```python
from build123d import *

# Parameters (mm, degrees)
SKETCH_1_R          = 9
EXTRUDE_1_DEPTH     = 2
SKETCH_2_R          = 6.78
EXTRUDE_2_DEPTH     = 11
SKETCH_3_R          = 9
EXTRUDE_3_DEPTH     = 2
SKETCH_4_R          = 2.5
CUT_EXTRUDE_1_DEPTH = 26


with BuildPart() as part:
    # 草图1 → 凸台-拉伸1 (new body)
    with BuildSketch(Plane(origin=(0, 0, 0), x_dir=(1, 0, 0), z_dir=(0, 1, 0))):
        with Locations(Location((0, 0, 0), (0, 0, 270))):
            Circle(SKETCH_1_R)
    extrude(amount=EXTRUDE_1_DEPTH)

    # 草图2 → 凸台-拉伸2 (add)
    with BuildSketch(Plane(origin=(0, 2, 0), x_dir=(1, 0, 0), z_dir=(0, 1, 0))):
        with Locations(Location((0, 0, 0), (0, 0, 270))):
            Circle(SKETCH_2_R)
    extrude(amount=EXTRUDE_2_DEPTH)

    # 草图3 → 凸台-拉伸3 (add)
    with BuildSketch(Plane(origin=(0, 13, 0), x_dir=(1, 0, 0), z_dir=(0, 1, 0))):
        with Locations(Location((0, 0, 0), (0, 0, 270))):
            Circle(SKETCH_3_R)
    extrude(amount=EXTRUDE_3_DEPTH)

    # 草图4 → 切除-拉伸1 (cut)
    with BuildSketch(Plane(origin=(0, 15, 0), x_dir=(1, 0, 0), z_dir=(0, 1, 0))):
        with Locations(Location((0, 0, 0), (0, 0, 270))):
            Circle(SKETCH_4_R)
    extrude(amount=-CUT_EXTRUDE_1_DEPTH, mode=Mode.SUBTRACT)


solid = part.part
```
Geometry check sheet. Reference: the model listing, model coordinates, mm. A direction names the side the tool comes from. Coordinates: 2 decimals unless noted, no trailing zeros. Order: outer loops, then holes, each group sorted by start corner. A loop starts at its lowest first (then second) coordinate and runs counter-clockwise, first axis right, second up. Notation, with made-up numbers: M 6,68 L 46,68 A9 cw 46,82 Z; hole C -26,64 d3. An arc over 180 degrees is marked long. Answer as a JSON object with one key per item and string values.
Q1. Scan lines: line 1 (Y direction, x = -3.5, z = 8.25); line 2 (X direction, y = 10, z = 0); line 3 (X direction, y = 10.5, z = -1.5). Record each from-to range of solid material in increasing order.
Results are:
{"line 1": "y = 0 to 2, 13 to 15", "line 2": "x = -6.78 to -2.5, 2.5 to 6.78", "line 3": "x = -6.61 to -2, 2 to 6.61"}
Q2. Tool access check on faces 1 (the flat face through (-2, 15, 2)), 2 (the flat face through (7, 2, 1)). Record the directions out of +Z, -Z, +X, -X, +Y, -Y that give a thin tool (end or side, any length) a straight path to the whole face; none if there is none.
Results are:
{"face 1": "+Z, -Z, +X, -X, +Y", "face 2": "none"}
Q3. Cross-section at A-A on x = 0. Record the cut outline in (y, z), and give its area (3 significant figures).
Results are:
{"outline": "M 0,-9 L 2,-9 L 2,-6.78 L 13,-6.78 L 13,-9 L 15,-9 L 15,-2.5 L 0,-2.5 Z; M 0,2.5 L 15,2.5 L 15,9 L 13,9 L 13,6.78 L 2,6.78 L 2,9 L 0,9 Z", "area": "146 mm²"}
Q4. Depth check by flat-ended pin: pin 1 Ø5 at (y, z) = (4, -5) entering from +X; pin 2 Ø2 at (x, y) = (2.5, 4) entering from -Z; pin 3 Ø5 at (y, z) = (5.5, 1) entering from +X. Enter the tip coordinate at first touch or a pass-through.
Results are:
{"pin 1": "stops at x = 8.29", "pin 2": "stops at z = -6.61", "pin 3": "stops at x = 6.78"}
Q5. Cross-section at B-B on z = 0. Record the cut outline in (x, y), and give its area (3 significant figures).
Results are:
{"outline": "M -9,0 L -2.5,0 L -2.5,15 L -9,15 L -9,13 L -6.78,13 L -6.78,2 L -9,2 Z; M 2.5,0 L 9,0 L 9,2 L 6.78,2 L 6.78,13 L 9,13 L 9,15 L 2.5,15 Z", "area": "146 mm²"}
Q6. Cross-section at C-C on y = 6.75. Record the cut outline in (x, z), and give its area (3 significant figures).
Results are:
{"outline": "C 0,0 d13.56; hole C 0,0 d5", "area": "125 mm²"}
Q7. Cross-section at D-D on z = -4.25. Record the cut outline in (x, y), and give its area (3 significant figures).
Results are:
{"outline": "M -7.93,0 L 7.93,0 L 7.93,2 L 5.28,2 L 5.28,13 L 7.93,13 L 7.93,15 L -7.93,15 L -7.93,13 L -5.28,13 L -5.28,2 L -7.93,2 Z", "area": "180 mm²"}
Q8. Release check for a two-part mould opening along X. For faces 3 (the flat face through (-2, 0, 2)), 4 (the cylindrical face through (-2.44, 7.6, -0.54)), 5 (the cylindrical face through (6.722, 7.423, -0.883)) record: released by +X, released by -X, zero draft, split by the parting line, or undercut.
Results are:
{"face 3": "zero draft", "face 4": "undercut", "face 5": "split by the parting line"}
